```python
from build123d import *

# Parameters (mm, degrees)
SKETCH_1_W          = 23.6
SKETCH_1_H          = 12
EXTRUDE_1_DEPTH     = 1.14
SKETCH_2_W          = 23.6
SKETCH_2_H          = 12
EXTRUDE_2_DEPTH     = 3.2
CUT_EXTRUDE_1_DEPTH = 18.380322206
EXTRUDE_3_DEPTH     = 3
EXTRUDE_4_DEPTH     = 3
EXTRUDE_START       = -8.34
SKETCH_6_W          = 4.5
SKETCH_6_H          = 18
EXTRUDE_6_DEPTH     = 6
SKETCH_9_W          = 18
SKETCH_9_H          = 6
EXTRUDE_8_DEPTH     = 4
SKETCH_11_W         = 8.5
SKETCH_11_H         = 18
EXTRUDE_11_DEPTH    = 2.34
SKETCH_13_W         = 18
SKETCH_13_H         = 6
EXTRUDE_12_DEPTH    = 2
SKETCH_14_W         = 18
SKETCH_14_H         = 8.34
EXTRUDE_13_DEPTH    = 8
SKETCH_15_W         = 6.5
SKETCH_15_H         = 18
EXTRUDE_14_DEPTH    = 2.34
SKETCH_12_R         = 1.65
CUT_EXTRUDE_2_DEPTH = 8.34
SKETCH_16_R         = 3
CUT_EXTRUDE_3_DEPTH = 3
SKETCH_17_R         = 9
SKETCH_17_R_2       = 6.303921286
EXTRUDE_15_DEPTH    = 2
SKETCH_18_R         = 9
EXTRUDE_16_DEPTH    = 1
CUT_EXTRUDE_START   = -10
SKETCH_19_R         = 1.65
CUT_EXTRUDE_4_DEPTH = 10
CUT_EXTRUDE_START_2 = -8.34
CUT_EXTRUDE_5_DEPTH = 8.34
CUT_EXTRUDE_6_DEPTH = 8.34
SKETCH_23_R         = 9
SKETCH_23_R_2       = 4
EXTRUDE_17_DEPTH    = 3.1


with BuildPart() as part:
    # 草图1 → 凸台-拉伸1 (new body)
    with BuildSketch(Plane(origin=(0, 0, 0), x_dir=(1, 0, 0), z_dir=(0, 1, 0))):
        Rectangle(SKETCH_1_W, SKETCH_1_H)
        with BuildLine():
            ThreePointArc((0.007454552, 3.287456445), (-3.58, 0), (0.007454552, -3.287456445))
            ThreePointArc((0.007454552, -3.287456445), (1.025918755, -3.405297551), (1.915651286, -3.91474027))
            ThreePointArc((1.915651286, -3.91474027), (11.52, 0), (1.915651286, 3.91474027))
            ThreePointArc((1.915651286, 3.91474027), (1.025918755, 3.405297551), (0.007454552, 3.287456445))
        make_face(mode=Mode.SUBTRACT)
    extrude(amount=-EXTRUDE_1_DEPTH)

    # 草图2 → 凸台-拉伸2 (add)
    with BuildSketch(Plane.XZ.offset(1.14)):
        Rectangle(SKETCH_2_W, SKETCH_2_H)
        with BuildLine():
            ThreePointArc((1.858985772, -4.210779433), (11.77, 0), (1.858985772, 4.210779433))
            ThreePointArc((1.858985772, 4.210779433), (1.095204485, 3.750394966), (0.20723472, 3.667778937))
            ThreePointArc((0.20723472, 3.667778937), (-3.98, 0), (0.20723472, -3.667778937))
            ThreePointArc((0.20723472, -3.667778937), (1.095204485, -3.750394966), (1.858985772, -4.210779433))
        make_face(mode=Mode.SUBTRACT)
    extrude(amount=EXTRUDE_2_DEPTH)

    # 草图3 → 切除-拉伸1 (cut, through all)
    with BuildSketch(Plane.XY.offset(6)):
        Polygon((-10.893933983, -4.233933983), (-11, -4.34), (11.220943823, -4.34), (11.220943823, -4.171669574), (10.902745772, -3.853471522), align=None)
    extrude(amount=-CUT_EXTRUDE_1_DEPTH, mode=Mode.SUBTRACT)

    # 草图4 → 凸台-拉伸3 (add)
    with BuildSketch(Plane.XY.offset(6)):
        Polygon((-11.8, -4.34), (-11.8, -8.34), (11.8, -8.34), (11.8, -4.34), (11.8, 0), (-11.8, 0), align=None)
    extrude(amount=EXTRUDE_3_DEPTH)

    # 草图5 → 凸台-拉伸4 (add)
    with BuildSketch(Plane(origin=(0, 0, -6), x_dir=(-1, 0, 0), z_dir=(0, 0, -1))):
        Polygon((11.8, -8.34), (-11.8, -8.34), (-11.8, -4.34), (-11.8, 0), (11.8, 0), (11.8, -4.34), align=None)
    extrude(amount=EXTRUDE_4_DEPTH)

    # 草图6 → 凸台-拉伸6 (add)
    with BuildSketch(Plane(origin=(0, 0, 0), x_dir=(1, 0, 0), z_dir=(0, 1, 0)).offset(EXTRUDE_START)):
        with Locations((14.05, 0)):
            Rectangle(SKETCH_6_W, SKETCH_6_H)
        with Locations((-14.05, 0)):
            Rectangle(SKETCH_6_W, SKETCH_6_H)
    extrude(amount=EXTRUDE_6_DEPTH)

    # 草图9 → 凸台-拉伸8 (add)
    with BuildSketch(Plane.ZY.offset(16.3)):
        with Locations((0, -5.34)):
            Rectangle(SKETCH_9_W, SKETCH_9_H)
    extrude(amount=EXTRUDE_8_DEPTH)

    # 草图11 → 凸台-拉伸11 (add)
    with BuildSketch(Plane(origin=(0, -2.34, 0), x_dir=(1, 0, 0), z_dir=(0, 1, 0))):
        with Locations((-16.05, 0)):
            Rectangle(SKETCH_11_W, SKETCH_11_H)
    extrude(amount=EXTRUDE_11_DEPTH)

    # 草图13 → 凸台-拉伸12 (add)
    with BuildSketch(Plane(origin=(16.3, 0, 0), x_dir=(0, 0, -1), z_dir=(1, 0, 0))):
        with Locations((0, -5.34)):
            Rectangle(SKETCH_13_W, SKETCH_13_H)
    extrude(amount=EXTRUDE_12_DEPTH)

    # 草图14 → 凸台-拉伸13 (add)
    with BuildSketch(Plane.ZY.offset(20.3)):
        with Locations((0, -4.17)):
            Rectangle(SKETCH_14_W, SKETCH_14_H)
    extrude(amount=EXTRUDE_13_DEPTH)

    # 草图15 → 凸台-拉伸14 (add)
    with BuildSketch(Plane(origin=(0, -2.34, 0), x_dir=(1, 0, 0), z_dir=(0, 1, 0))):
        with Locations((15.05, 0)):
            Rectangle(SKETCH_15_W, SKETCH_15_H)
    extrude(amount=EXTRUDE_14_DEPTH)

    # 草图12 → 切除-拉伸2 (cut)
    with BuildSketch(Plane(origin=(0, 0, 0), x_dir=(1, 0, 0), z_dir=(0, 1, 0))):
        with Locations(Location((-15.61, 0, 0), (0, 0, 270))):
            Circle(SKETCH_12_R)
    extrude(amount=-CUT_EXTRUDE_2_DEPTH, mode=Mode.SUBTRACT)

    # 草图16 → 切除-拉伸3 (cut)
    with BuildSketch(Plane.XZ.offset(8.34)):
        with Locations(Location((-15.61, 0, 0), (0, 0, 270))):
            Circle(SKETCH_16_R)
    extrude(amount=-CUT_EXTRUDE_3_DEPTH, mode=Mode.SUBTRACT)

    # 草图17 → 凸台-拉伸15 (add)
    with BuildSketch(Plane(origin=(0, 0, 0), x_dir=(1, 0, 0), z_dir=(0, 1, 0))):
        with Locations(Location((5.92, 0, 0), (0, 0, 270))):
            Circle(SKETCH_17_R)
        with Locations(Location((5.92, 0, 0), (0, 0, 148.458888043))):
            Circle(SKETCH_17_R_2, mode=Mode.SUBTRACT)
    extrude(amount=EXTRUDE_15_DEPTH)

    # 草图18 → 凸台-拉伸16 (add)
    with BuildSketch(Plane(origin=(0, 0, 0), x_dir=(1, 0, 0), z_dir=(0, 1, 0))):
        with Locations(Location((-15.61, 0, 0), (0, 0, 270))):
            Circle(SKETCH_18_R)
    extrude(amount=EXTRUDE_16_DEPTH)

    # 草图19 → 切除-拉伸4 (cut)
    with BuildSketch(Plane.XZ.offset(CUT_EXTRUDE_START)):
        with Locations(Location((-15.61, 0, 0), (0, 0, 90))):
            Circle(SKETCH_19_R)
    extrude(amount=CUT_EXTRUDE_4_DEPTH, mode=Mode.SUBTRACT)

    # 草图20 → 切除-拉伸5 (cut)
    with BuildSketch(Plane(origin=(0, 0, 0), x_dir=(1, 0, 0), z_dir=(0, 1, 0)).offset(CUT_EXTRUDE_START_2)):
        with BuildLine():
            Line((-15.61, -9), (-28.3, -9))
            Line((-28.3, -9), (-28.3, 9))
            Line((-28.3, 9), (-15.61, 9))
            ThreePointArc((-15.61, 9), (-24.61, 0), (-15.61, -9))
        make_face()
    extrude(amount=CUT_EXTRUDE_5_DEPTH, mode=Mode.SUBTRACT)

    # 草图21 → 切除-拉伸6 (cut)
    with BuildSketch(Plane(origin=(0, 0, 0), x_dir=(1, 0, 0), z_dir=(0, 1, 0))):
        with BuildLine():
            ThreePointArc((9.3, 9), (15.663961016, 6.363961045), (18.3, 4.1e-08))
            Line((18.3, 4.1e-08), (18.3, 9))
            Line((18.3, 9), (12.11, 9))
            Line((12.11, 9), (9.3, 9))
        make_face()
        with BuildLine():
            ThreePointArc((18.3, 4.1e-08), (15.663961045, -6.363961016), (9.3, -9))
            Line((9.3, -9), (18.3, -9))
            Line((18.3, -9), (18.3, 4.1e-08))
        make_face()
    extrude(amount=-CUT_EXTRUDE_6_DEPTH, mode=Mode.SUBTRACT)

    # 草图23 → 凸台-拉伸17 (add)
    with BuildSketch(Plane(origin=(0, 1, 0), x_dir=(1, 0, 0), z_dir=(0, 1, 0))):
        with Locations(Location((-15.61, 0, 0), (0, 0, 270))):
            Circle(SKETCH_23_R)
        with Locations(Location((-15.61, 0, 0), (0, 0, 90))):
            Circle(SKETCH_23_R_2, mode=Mode.SUBTRACT)
    extrude(amount=EXTRUDE_17_DEPTH)


solid = part.part
```
CAD build for the part. Positions are in the model's coordinates, mm. A direction names the side the tool comes from. Give positions to 0.01 mm unless a question says otherwise; leave off trailing zeros. Write each loop counter-clockwise with the first axis right and the second up, starting at its lowest first coordinate (ties: lowest second). Pieces come first, ordered by that corner, then holes. Notation, with made-up numbers: (89, -17) -> (117, -17) arc R35 ccw to (117, 18) -> close; hole circle Ø1 at (88.5, 30.25). An arc over 180 degrees is marked (long way). Write each question's results on one line, items separated by ' | '.
1. Cut at C-C, the plane y = -0.5. Write the cut outline in (x, z).
Geometry check:
outline: (-15.61, -9) -> (9.3, -9) arc R9 ccw to (9.3, 9) -> (-15.61, 9) arc R9 ccw to start; hole circle Ø3.3 at (-15.61, 0); hole (0.01, -3.29) arc R2.55 cw to (1.92, -3.91) arc R5.6 ccw (long way) to (1.92, 3.91) arc R2.55 cw to (0.01, 3.29) arc R3.3 ccw (long way) to start
2. Which spindle directions (+Z, -Z, +X, -X, +Y, -Y) get a long thin tool onto all of the face, cutting with end or side? Do faces 1 (the flat face through (-16, 1, 2)), 2 (the flat face through (-3, -4, 9)), 3 (the flat face through (0, -6, 6)). Say none if no direction does.
Geometry check:
face 1: +Y | face 2: +Z, +X, -X, +Y, -Y | face 3: -Y
3. Drop flat-ended pins along their axis: P1, Ø0.5, axis at x = 11.5, z = -2, coming from the -Y side; P2, Ø2, axis at x = -9.5, z = 0.5, coming from the -Y side; P3, Ø2, axis at y = -5.5, z = -2.5, coming from the -X side. Give the stop position or say it passes through.
Geometry check:
P1: y = -4.34 | P2: y = -4.23 | P3: x = -24.48
4. Cut at B-B, the plane x = -9.5. Write the cut outline in (y, z), then the cut area to 3 significant figures.
Geometry check:
outline: (-8.34, -9) -> (0, -9) -> (0, -6.61) -> (4.1, -6.61) -> (4.1, 6.61) -> (0, 6.61) -> (0, 9) -> (-8.34, 9) -> (-8.34, 6) -> (-4.21, 6) -> (-4.21, -6) -> (-8.34, -6) -> close | area: 155 mm²
5. Two-plate mould, pull along X, no slides. Class faces 4 (the flat face through (8.05, 2, -6.13)), 5 (the flat face through (-1, 0, 0)): pulls with the +X half, pulls with the -X half, needs draft (parallel to the pull), parting line crosses it, or undercut.
Geometry check:
face 4: needs draft | face 5: undercut
6. Wall check: probe 1 along X at (y, z) = (-3.25, 0); probe 2 along X at (y, z) = (0.55, 0); probe 3 along Z at (x, y) = (5, -7). Give the ranges that are in metal, low to high. Write a range as [from, to].
Geometry check:
probe 1: [-24.61, -17.26], [-13.96, -3.98], [11.77, 18.3] | probe 2: [-24.61, -17.26], [-13.96, -6.61], [-3.08, -0.38], [12.22, 14.92] | probe 3: [-9, -6], [6, 9]
7. Cut at D-D, the plane x = -1.5. Write the cut outline in (y, z), then the cut area to 3 significant figures.
Geometry check:
outline: (-8.34, -9) -> (0, -9) -> (0, -5.09) -> (2, -5.09) -> (2, 5.09) -> (0, 5.09) -> (0, 9) -> (-8.34, 9) -> (-8.34, 6) -> (-4.07, 6) -> (-4.07, 3.49) -> (-1.14, 3.49) -> (-1.14, 3.07) -> (0, 3.07) -> (0, -3.07) -> (-1.14, -3.07) -> (-1.14, -3.49) -> (-4.07, -3.49) -> (-4.07, -6) -> (-8.34, -6) -> close | area: 91.8 mm²
8. Cut at A-A, the plane y = -7. Write the cut outline in (x, z).
Geometry check:
outline: (-15.61, -9) -> (9.3, -9) arc R9 ccw to (9.3, 9) -> (-15.61, 9) arc R9 ccw to start; hole circle Ø6 at (-15.61, 0); hole (-11.8, -6) -> (11.8, -6) -> (11.8, 6) -> (-11.8, 6) -> close
